from build123d import *

# Parameters (mm, degrees)
SKETCH1_R           = 25
BOSS_EXTRUDE1_DEPTH = 60
CUT_EXTRUDE3_DEPTH  = 60
SKETCH2_4_R         = 25
BOSS_EXTRUDE2_DEPTH = 120
FILLET1_R           = 12


with BuildPart() as part:
    # Sketch1 → Boss-Extrude1 (new body)
    with BuildSketch(Plane.YZ):
        with BuildLine():
            Line((60, 30), (180, 30))
            Line((180, 30), (180, -30))
            Line((180, -30), (60, -30))
            ThreePointArc((60, -30), (44.188611699, -32.565835097), (30, -40))
            ThreePointArc((30, -40), (-50, 0), (30, 40))
            ThreePointArc((30, 40), (44.188611699, 32.565835097), (60, 30))
        make_face()
        with Locations(Location((0, 0, 0), (0, 0, 270))):
            Circle(SKETCH1_R, mode=Mode.SUBTRACT)
    extrude(amount=BOSS_EXTRUDE1_DEPTH)

    # Sketch2 → Cut-Extrude3 (cut)
    with BuildSketch(Plane(origin=(0, 180, 0), x_dir=(-1, 0, 0), z_dir=(0, 1, 0))):
        Polygon((-60, 11.94), (-41.94, 30), (-60, 30), align=None)
        Polygon((0, 30), (-18.06, 30), (0, 11.94), align=None)
        Polygon((0, -30), (0, -11.94), (-18.06, -30), align=None)
        Polygon((-41.94, -30), (-60, -11.94), (-60, -30), align=None)
    extrude(amount=-CUT_EXTRUDE3_DEPTH, mode=Mode.SUBTRACT)

    # Sketch2_4 → Boss-Extrude2 (add)
    with BuildSketch(Plane(origin=(0, 180, 0), x_dir=(-1, 0, 0), z_dir=(0, 1, 0))):
        with Locations(Location((-30, 0, 0), (0, 0, 90))):
            Circle(SKETCH2_4_R)
    extrude(amount=BOSS_EXTRUDE2_DEPTH)

    # Fillet1
    fillet1_edges = [part.edges().sort_by_distance(p)[0] for p in [
        (50.97, 120, -20.97),
        (9.03, 120, -20.97),
        (9.03, 120, 20.97),
        (50.97, 120, 20.97),
    ]]
    fillet(fillet1_edges, radius=FILLET1_R)


solid = part.part
Source: CAD feature listing. Evaluate the final solid. Frame: model axes, mm. A direction names the side the tool comes from. Round coordinates to 2 decimals unless told otherwise and drop trailing zeros. Loops run counter-clockwise (first coordinate to the right, second up) from the corner with the lowest first, then second, coordinate; pieces in that order, holes last. Notation, with made-up numbers: (22.25, -22) - (31.25, -22) arc R25 ccw to (31.25, 2) - close; hole circle Ø3 at (77, -21). An arc over 180 degrees is marked (long way). Write item = value, one per line. Start each with the question number.
Item 1: Mould query, pull axis Y, two halves, no side actions, for faces 6 (the face through (52.578, 125.226, -22.325)), 7 (the face through (30, 106, 30)), 8 (the face through (29.58, 7.509, -23.846)). Classes: released by +Y, released by -Y, zero draft, split by the parting line, or undercut.
Item 2: Section query A-A on y = 0. Output: boundary loops of the cut face in (x, z), plus the area to 3 significant figures.
Item 3: Material intervals for line 1 (Z direction, x = 35.5, y = -0.5) (1 decimal); line 2 (Y direction, x = 15, z = 0); line 3 (Z direction, x = 42, y = 168.5), sorted ascending.
Item 4: Section query C-C on z = 0. Output: boundary loops of the cut face in (x, y), plus the area to 3 significant figures.
Item 5: Section query B-B on x = 30. Output: boundary loops of the cut face in (y, z), plus the area to 3 significant figures.
Item 6: Reachability of faces 1 (the face through (30, 108, -30)), 2 (the face through (48, 180, 18)), 3 (the face through (50.84, 156.34, -21.1)), 4 (the face through (8.9, 156.34, -20.84)), 5 (the face through (51.1, 156.34, 20.84)) from +Z, -Z, +X, -X, +Y, -Y: full face, straight path, thin tool, end or side. Return the list, or none.
Item 7: Section query D-D on y = 109.5. Output: boundary loops of the cut face in (x, z).
Item 8: First-contact query: pin 1 Ø12 at (x, z) = (22, 5) entering from -Y; pin 2 Ø1 at (x, y) = (11, 182) entering from +Z; pin 3 Ø0.5 at (x, z) = (0.5, -29) entering from +Y; pin 4 Ø2 at (x, y) = (21.5, 106.5) entering from -Z. Flat tips, straight axial feed; report the tip coordinate or a pass-through.
Results list:
q1.face_6 = released by +Y
q1.face_7 = zero draft
q1.face_8 = undercut
q2.outline = (0, -50) - (60, -50) - (60, -25) - (0, -25) - close; (0, 25) - (60, 25) - (60, 50) - (0, 50) - close
q2.area = 3,000 mm²
q3.line_1 = -50 to -25, 25 to 50
q3.line_2 = -50 to -25, 25 to 300
q3.line_3 = -29.94 to 29.94
q4.outline = (0, -50) - (60, -50) - (60, -25) - (0, -25) - close; (0, 25) - (60, 25) - (60, 180) - (55, 180) - (55, 300) - (5, 300) - (5, 180) - (0, 180) - close
q4.area = 16,800 mm²
q5.outline = (30, -40) arc R50 cw to (60, -30) - (180, -30) - (180, -25) - (300, -25) - (300, 25) - (180, 25) - (180, 30) - (60, 30) arc R50 cw to (30, 40) arc R50 ccw (long way) to start; hole circle Ø50 at (0, 0)
q5.area = 20,000 mm²
q6.face_1 = -Z, +X, -X, +Y
q6.face_2 = +Y
q6.face_3 = -Z, +X, +Y
q6.face_4 = -Z, -X, +Y
q6.face_5 = +Z, +X, +Y
q7.outline = (0, -30) - (60, -30) - (60, 30) - (0, 30) - close
q8.pin_1 = -50
q8.pin_2 = 16.82
q8.pin_3 = 120.01
q8.pin_4 = -30
